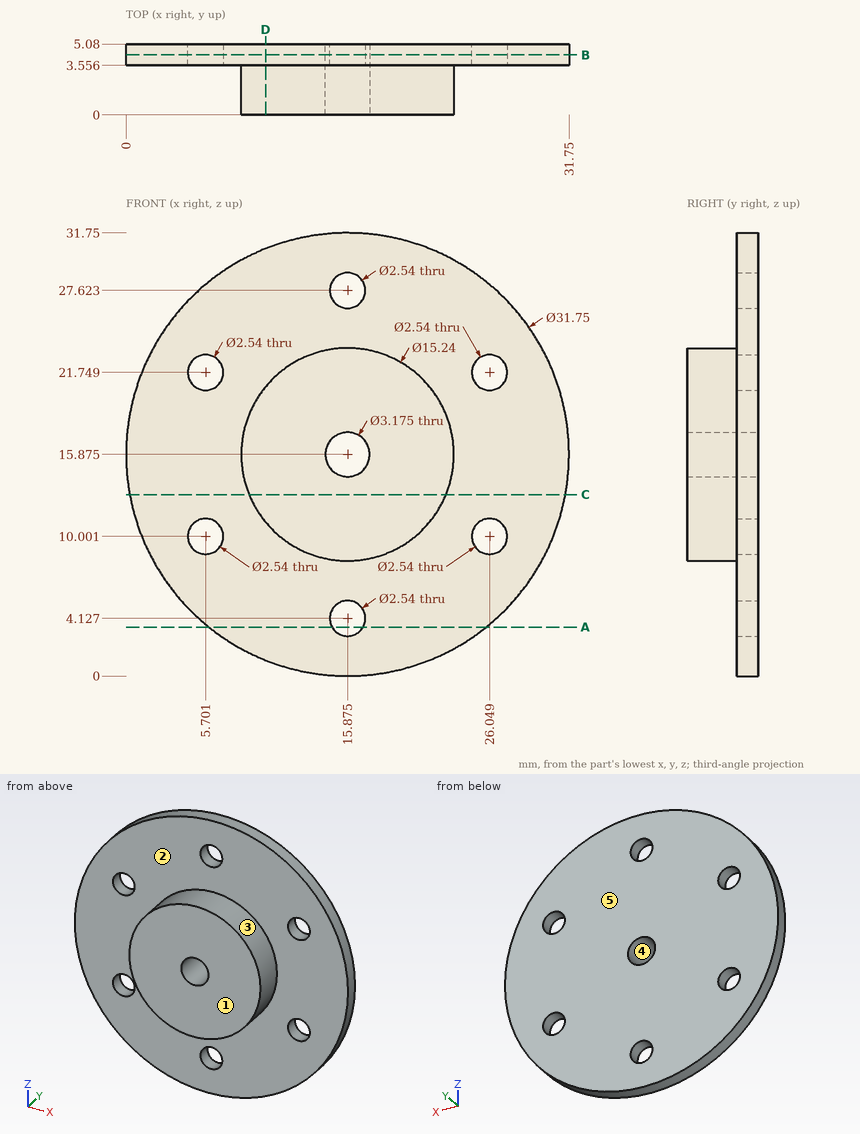
Answer from the drawing. Dimensions are ordinates in mm from the lowest x, y and z of the part. A direction names the side the tool comes from. Coordinates: 2 decimals unless noted, no trailing zeros. Write each loop counter-clockwise with the first axis right and the second up, starting at its lowest first coordinate (ties: lowest second). Pieces come first, ordered by that corner, then holes. Notation, with made-up numbers: M 37,-19 L 69,-19 A20 cw 69,-7 Z; hole C -18.75,-24.75 d3. An arc over 180 degrees is marked long. Put each result on its own line as item: value. Start each with the question number.
1. A cutting plane is placed at C-C on z = 13. Write down the section's boundary in (x, y) (1 decimal).
2. A cutting plane is placed at A-A on z = 3.5. Write down the section's boundary in (x, y) (1 decimal).
3. Consider line 1 (Y direction, x = 30.5, z = 17) (1 decimal); line 2 (X direction, y = 4.95, z = 9) (1 decimal); line 3 (X direction, y = 2.65, z = 14.5) (1 decimal). Determine where each line is inside the solid, lowest interval first. Write a range as from..to.
4. For a pull along X with two mould halves and no side action, classify the marked faces 3, 4 and 5 as pulls with the +X half, pulls with the -X half, needs draft (parallel to the pull), parting line crosses it, or undercut.
5. Which of the six approach directions +Z, -Z, +X, -X, +Y, -Y give full straight-line access (tool end or side, diameter ignored) to the marked faces 1 and 2?
6. A cutting plane is placed at B-B on y = 4.3. Count the separate pieces of the cut face and the enclosed holes in it.
7. A cutting plane is placed at D-D on x = 10. Write down the section's boundary in (y, z) (1 decimal).
8. Flat-ended cylindrical pins translate along their axes: P1, Ø3, axis at y = 3.5, z = 8, coming from the +X side; P2, Ø4, axis at x = 25, z = 9.5, coming from the -Y side; P3, Ø3.5, axis at x = 15.875, z = 15.875, coming from the -Y side; P4, Ø3, axis at y = 1.5, z = 19.5, coming from the -X side. Find the tip coordinate at first contact, or state that the pin passes through.
Resolved:
1. outline: M 0.3,3.6 L 8.8,3.6 L 8.8,0 L 22.9,0 L 22.9,3.6 L 31.5,3.6 L 31.5,5.1 L 0.3,5.1 Z
2. outline: M 5.9,3.6 L 14.8,3.6 L 14.8,5.1 L 5.9,5.1 Z; M 17,3.6 L 25.8,3.6 L 25.8,5.1 L 17,5.1 Z
3. line 1: y = 3.6..5.1
3. line 2: x = 1.6..4.9, 6.5..25.3, 26.8..30.2
3. line 3: x = 8.4..15.1, 16.7..23.4
4. face 3: parting line crosses it
4. face 4: undercut
4. face 5: needs draft
5. face 1: +Z, -Z, +X, -X, -Y
5. face 2: -Y
6. separate pieces: 1
6. enclosed holes: 7
7. outline: M 0,11 L 3.6,11 L 3.6,1.1 L 5.1,1.1 L 5.1,30.6 L 3.6,30.6 L 3.6,20.7 L 0,20.7 Z
8. P1: stops at x = 30.41
8. P2: stops at y = 3.56
8. P3: stops at y = 0
8. P4: stops at x = 8.56
